from build123d import *

# Parameters (mm, degrees)
SKETCH1_W           = 431.8
SKETCH1_H           = 557.4328891
BOSS_EXTRUDE1_DEPTH = 40
FILLET1_START       = -215.9
FILLET1_DEPTH       = 431.8
FILLET1_START_2     = -280
FILLET1_2_DEPTH     = 560


with BuildPart() as part:
    # Sketch1 → Boss-Extrude1 (new body)
    with BuildSketch(Plane(origin=(0, 0, 0), x_dir=(1, 0, 0), z_dir=(0, 1, 0))):
        Rectangle(SKETCH1_W, SKETCH1_H)
    extrude(amount=BOSS_EXTRUDE1_DEPTH)

    # Fillet1: read off the stored shape, not the designer's step
    # Fillet1 outline → Fillet1 (cut)
    with BuildSketch(Plane.YZ.offset(FILLET1_START)):
        with BuildLine():
            Line((40, -278.71644455), (40, -258.71644455))
            ThreePointArc((40, -258.71644455), (34.142135624, -272.858580174), (20, -278.71644455))
            Line((20, -278.71644455), (40, -278.71644455))
        make_face()
        with BuildLine():
            ThreePointArc((20, 278.71644455), (34.142135624, 272.858580174), (40, 258.71644455))
            Line((40, 258.71644455), (40, 278.71644455))
            Line((40, 278.71644455), (20, 278.71644455))
        make_face()
    extrude(amount=FILLET1_DEPTH, mode=Mode.SUBTRACT)

    # Fillet1 2 outline → Fillet1 2 (cut)
    with BuildSketch(Plane.XY.offset(FILLET1_START_2)):
        with BuildLine():
            Line((215.9, 40), (195.9, 40))
            ThreePointArc((195.9, 40), (210.042135624, 34.142135624), (215.9, 20))
            Line((215.9, 20), (215.9, 40))
        make_face()
        with BuildLine():
            ThreePointArc((-215.9, 20), (-210.042135624, 34.142135624), (-195.9, 40))
            Line((-195.9, 40), (-215.9, 40))
            Line((-215.9, 40), (-215.9, 20))
        make_face()
    extrude(amount=FILLET1_2_DEPTH, mode=Mode.SUBTRACT)


solid = part.part
Work out the finished part from the listing and answer in its coordinate system (mm). Coordinates: 2 decimals unless noted, no trailing zeros. Write each loop counter-clockwise with the first axis right and the second up, starting at its lowest first coordinate (ties: lowest second). Pieces come first, ordered by that corner, then holes. Notation, with made-up numbers: M 60,80 L 113,80 A20 ccw 113,98 Z; hole C 36.25,54 d9. An arc over 180 degrees is marked long. Answer as CSV lines item,"result". Start each with the question number.
Item 1: Consider L1, parallel to X at y = 21, z = -144.5; L2, parallel to Z at x = -179, y = 20.5; L3, parallel to Z at x = -161, y = 32. Determine where each line is inside the solid, lowest interval first.
Item 2: Flat-ended cylindrical pins translate along their axes: P1, Ø8, axis at y = 28.5, z = 203, coming from the -X side; P2, Ø3, axis at y = 36, z = -95.5, coming from the +X side (3 decimals); P3, Ø1, axis at x = -37.5, y = 32.5, coming from the +Z side. Find the tip coordinate at first contact, or state that the pin passes through.
Item 3: Section A-A on y = 33.5 is taken. Write down the section's boundary in (x, z).
Checks:
1,L1,"x = -215.87 to 215.87"
1,L2,"z = -278.71 to 278.71"
1,L3,"z = -274.72 to 274.72"
2,P1,"stops at x = -215.39"
2,P2,"stops at x = 209.675"
2,P3,"stops at z = 274.72"
3,outline,"M -210.66,-273.47 L 210.66,-273.47 L 210.66,273.47 L -210.66,273.47 Z"
